Can you work these out from the model? Positions are in its coordinate system, mm. A direction names the side the tool comes from. Give positions to 0.01 mm unless a question says otherwise; leave off trailing zeros. Loops run counter-clockwise (first coordinate to the right, second up) from the corner with the lowest first, then second, coordinate; pieces in that order, holes last. Notation, with made-up numbers: (78.25, -23.75) - (110.25, -23.75) arc R17 cw to (110.25, -4.75) - close; hole circle Ø2 at (79, 88). An arc over 180 degrees is marked (long way). Answer in a Markdown table with one row per item.
from build123d import *

# Parameters (mm, degrees)
SKETCH1_R           = 16.5
BOSS_EXTRUDE1_DEPTH = 22.5
SKETCH2_R           = 18.5
BOSS_EXTRUDE2_DEPTH = 23
SKETCH3_R           = 6
BOSS_EXTRUDE3_DEPTH = 6
SKETCH4_R           = 3
BOSS_EXTRUDE4_DEPTH = 25
FILLET4_R           = 0.5
FILLET5_R           = 0.5
FILLET6_R           = 0.5
FILLET7_R           = 0.5
SKETCH9_R           = 5
BOSS_EXTRUDE5_DEPTH = 2
SKETCH10_R          = 1
BOSS_EXTRUDE6_DEPTH = 1
SKETCH11_W          = 13.803464896
SKETCH11_H          = 3.909651907
SKETCH11_W_2        = 12.803464896
SKETCH11_H_2        = 2.909651907
BOSS_EXTRUDE7_DEPTH = 5
SKETCH12_W          = 2
SKETCH12_H          = 1
CUT_EXTRUDE5_DEPTH  = 2
SKETCH13_W          = 0.5
SKETCH13_H          = 0.5
BOSS_EXTRUDE8_DEPTH = 4


with BuildPart() as part:
    # Sketch1 → Boss-Extrude1 (new body)
    with BuildSketch(Plane(origin=(0, 0, 0), x_dir=(1, 0, 0), z_dir=(0, 1, 0))):
        with Locations(Location((0, 0, 0), (0, 0, 90))):
            Circle(SKETCH1_R)
    extrude(amount=BOSS_EXTRUDE1_DEPTH)

    # Sketch2 → Boss-Extrude2 (add)
    with BuildSketch(Plane(origin=(0, 22.5, 0), x_dir=(1, 0, 0), z_dir=(0, 1, 0))):
        with Locations(Location((0, 0, 0), (0, 0, 270))):
            Circle(SKETCH2_R)
    extrude(amount=BOSS_EXTRUDE2_DEPTH)

    # Sketch3 → Boss-Extrude3 (add)
    with BuildSketch(Plane(origin=(0, 45.5, 0), x_dir=(1, 0, 0), z_dir=(0, 1, 0))):
        with Locations(Location((0, 0.01, 0), (0, 0, 270))):
            Circle(SKETCH3_R)
    extrude(amount=BOSS_EXTRUDE3_DEPTH)

    # Sketch4 → Boss-Extrude4 (add)
    with BuildSketch(Plane(origin=(0, 51.5, 0), x_dir=(1, 0, 0), z_dir=(0, 1, 0))):
        with Locations(Location((0, 0.01, 0), (0, 0, 270))):
            Circle(SKETCH4_R)
    extrude(amount=BOSS_EXTRUDE4_DEPTH)

    # Fillet4
    fillet4_edges = [part.edges().sort_by_distance(p)[0] for p in [
        (0, 22.5, -18.5),
    ]]
    fillet(fillet4_edges, radius=FILLET4_R)

    # Fillet5
    fillet5_edges = [part.edges().sort_by_distance(p)[0] for p in [
        (0, 0, 16.5),
    ]]
    fillet(fillet5_edges, radius=FILLET5_R)

    # Fillet6
    fillet6_edges = [part.edges().sort_by_distance(p)[0] for p in [
        (0, 45.5, -18.5),
    ]]
    fillet(fillet6_edges, radius=FILLET6_R)

    # Fillet7
    fillet7_edges = [part.edges().sort_by_distance(p)[0] for p in [
        (0, 51.5, -6.01),
    ]]
    fillet(fillet7_edges, radius=FILLET7_R)

    # Sketch9 → Boss-Extrude5 (add)
    with BuildSketch(Plane.XZ):
        with Locations(Location((0, 0, 0), (0, 0, 90))):
            Circle(SKETCH9_R)
    extrude(amount=BOSS_EXTRUDE5_DEPTH)

    # Sketch10 → Boss-Extrude6 (add)
    with BuildSketch(Plane.XZ.offset(2)):
        with Locations(Location((0, 0, 0), (0, 0, 270))):
            Circle(SKETCH10_R)
    extrude(amount=BOSS_EXTRUDE6_DEPTH)

    # Sketch11 → Boss-Extrude7 (add)
    with BuildSketch(Plane.XZ):
        with Locations((0, 10.224361626)):
            Rectangle(SKETCH11_W, SKETCH11_H)
        with Locations((0, 10.224361626)):
            Rectangle(SKETCH11_W_2, SKETCH11_H_2, mode=Mode.SUBTRACT)
    extrude(amount=BOSS_EXTRUDE7_DEPTH)

    # Sketch12 → Cut-Extrude5 (cut)
    with BuildSketch(Plane.XY.offset(12.179187579)):
        with Locations((-3.901732448, -4.5)):
            Rectangle(SKETCH12_W, SKETCH12_H)
        with Locations((3.901732448, -4.5)):
            Rectangle(SKETCH12_W, SKETCH12_H)
    extrude(amount=-CUT_EXTRUDE5_DEPTH, mode=Mode.SUBTRACT)

    # Sketch13 → Boss-Extrude8 (add)
    with BuildSketch(Plane.XZ):
        with Locations((-4.651732448, 10.224361626)):
            Rectangle(SKETCH13_W, SKETCH13_H)
        with Locations((-1.651732448, 10.224361626)):
            Rectangle(SKETCH13_W, SKETCH13_H)
        with Locations((1.348267552, 10.224361626)):
            Rectangle(SKETCH13_W, SKETCH13_H)
        with Locations((4.348267552, 10.224361626)):
            Rectangle(SKETCH13_W, SKETCH13_H)
    extrude(amount=BOSS_EXTRUDE8_DEPTH)


solid = part.part
Q1. For pin 1 (1.5 mm diameter, centred on x = -12, z = -12.5, fed in from -Y); pin 2 (0.6 mm diameter, centred on y = -2, z = 10, fed in from -X); pin 3 (1 mm diameter, centred on x = -0.5, z = 0.5, fed in from -Y), each with a flat end and sliding along its axis, tell me the tip position at first contact or that it passes through.
Checked values:
| item | result |
|---|---|
| pin 1 | stops at y = 22.5 |
| pin 2 | stops at x = -6.9 |
| pin 3 | stops at y = -3 |
Q2. Imagine slicing it at A-A, the plane y = 39. Write out the boundary of the cut face in (x, z).
Checked values:
| item | result |
|---|---|
| outline | circle Ø37 at (0, 0) |
Q3. If we mould it in two halves opening along X, with no side actions, what happens to faces 4 (the face through (-7.086, 33.846, 17.089)), 5 (the face through (-6.902, -2, 10)), 6 (the face through (0, 76.5, 0)), 7 (the face through (6.402, -2, 10))? For each: released by +X, released by -X, zero draft, split by the parting line, or undercut.
Checked values:
| item | result |
|---|---|
| face 4 | split by the parting line |
| face 5 | released by -X |
| face 6 | zero draft |
| face 7 | undercut |
Q4. If I drill on line 1 (X direction, y = 20.5, z = -0.5); line 2 (Y direction, x = -4.5, z = -14); line 3 (Z direction, x = 8, y = 31), over which ranges is the centre line in solid material (lowest first)? Write a range as [from, to].
Checked values:
| item | result |
|---|---|
| line 1 | x = [-16.49, 16.49] |
| line 2 | y = [0, 45.5] |
| line 3 | z = [-16.68, 16.68] |
Q5. On a 3-axis mill with a long thin cutter (end or side, diameter ignored), from which of +Z, -Z, +X, -X, +Y, -Y can I reach the whole of each face in a straight line? I mean faces 1 (the face through (0, -2, 8.77)), 2 (the face through (0, -3, 0)), 3 (the face through (6.902, -2, 10)). Say none if no direction works.
Checked values:
| item | result |
|---|---|
| face 1 | -Y |
| face 2 | -Z, +X, -X, -Y |
| face 3 | +Z, -Z, +X, -Y |
